Source: CAD feature listing. Evaluate the final solid. Frame: model axes, mm. A direction names the side the tool comes from. Round coordinates to 2 decimals unless told otherwise and drop trailing zeros. Order: outer loops, then holes, each group sorted by start corner. A loop starts at its lowest first (then second) coordinate and runs counter-clockwise, first axis right, second up. Notation, with made-up numbers: (44.5, -5) - (79.5, -5) arc R11 ccw to (79.5, 16) - close; hole circle Ø7 at (-5, -31). An arc over 180 degrees is marked (long way). Use one line per item in the form item = value. Start each with the question number.
Q1. Set-up query: faces 1 (the flat face through (-90, 0, -70)), 2 (the cylindrical face through (-70.02, -0.88, -62.4)), 3 (the cylindrical face through (-109.98, -0.88, 2.39)). Return all of +Z, -Z, +X, -X, +Y, -Y with unobstructed straight access to the full face (end or side cutting, diameter ignored); none if empty.
Q2. Cut plane A-A, the plane x = -90. Return the cut outline in (y, z), and give its area (3 significant figures).
Q3. Cut plane C-C, the plane z = -44.5. Return the cut outline in (x, y), and give its area (3 significant figures).
Q4. Cut plane B-B, the plane y = 0. Return the cut outline in (x, z), and give its area (3 significant figures).
Q5. Cut plane D-D, the plane z = -7.5. Return the cut outline in (x, y).
Q6. Pin query (flat end, axial travel): pin 1 Ø10 at (y, z) = (5, -40) entering from +X; pin 2 Ø10 at (x, z) = (-116.5, -36) entering from +Y; pin 3 Ø5 at (y, z) = (14.5, -40) entering from +X; pin 4 Ø8 at (x, y) = (-152, -29.5) entering from -Z. Return the tip coordinate at first contact, or that it passes through.
Q7. Ray query, line 1 (Z direction, x = -66, y = -24); line 2 (Y direction, x = -119, z = -26); line 3 (X direction, y = 74, z = -24.5). Return the intervals inside material, ascending. Write a range as [from, to].
Autodesk Inventor part; units mm, degrees
ref_plane "YZ Plane" through (0, 0, 0) normal (1, 0, 0) x (0, 1, 0)
ref_plane "XZ Plane" through (0, 0, 0) normal (0, 1, 0) x (-1, 0, 0)
ref_plane "XY Plane" through (0, 0, 0) normal (0, 0, 1) x (1, 0, 0)
ref_plane "РабПлоскость3" through (0.0801, 60, -30) normal (0, 0, 1) x (1, 0, 0)
sketch "Эскиз1" plane through (0.0801, 60, -30) normal (0, 0, 1) x (1, 0, 0)
  line L0 (-0.0801, -60) -> (-90.0801, -60)
  circle A0 centre (-90.0801, -60) radius 87.5
  dimension "d0" = 90
  dimension "d1" = 175
extrude "Выдавливание1" add sketch "Эскиз1" along normal mid plane 50
sketch "Эскиз2" plane through (-90, 0, -5) normal (0, 0, 1) x (1, 0, 0)
  circle A0 centre (0, 0) radius 20
  point P0 (90, 0)
  dimension "d4" = 40
extrude "Выдавливание2" add sketch "Эскиз2" along normal blind 15
sketch "Эскиз3" plane through (-90, 0, -55) normal (0, 0, -1) x (-1, 0, 0)
  circle A0 centre (0, 0) radius 20
  circle A1 centre (0, 0) radius 20
  point P0 (-90, 0)
  dimension "d7" = 40
extrude "Выдавливание3" add sketch "Эскиз3" along normal blind 15
fillet "Сопряжение1" radius 5 1 edges at (-177.5, 0, -5)
fillet "Сопряжение2" radius 5 1 edges at (-177.5, 0, -55)
properties part number "Колесо"
Completed:
q1.face_1 = -Z, +X, -X, +Y, -Y
q1.face_2 = -Z
q1.face_3 = +Z
q2.outline = (-87.5, -50) arc R5 ccw to (-82.5, -55) - (-20, -55) - (-20, -70) - (20, -70) - (20, -55) - (82.5, -55) arc R5 ccw to (87.5, -50) - (87.5, -10) arc R5 ccw to (82.5, -5) - (20, -5) - (20, 10) - (-20, 10) - (-20, -5) - (-82.5, -5) arc R5 ccw to (-87.5, -10) - close
q2.area = 9,930 mm2
q3.outline = circle Ø175 at (-90, 0)
q3.area = 24,100 mm2
q4.outline = (-177.5, -50) arc R5 ccw to (-172.5, -55) - (-110, -55) - (-110, -70) - (-70, -70) - (-70, -55) - (-7.5, -55) arc R5 ccw to (-2.5, -50) - (-2.5, -10) arc R5 ccw to (-7.5, -5) - (-70, -5) - (-70, 10) - (-110, 10) - (-110, -5) - (-172.5, -5) arc R5 ccw to (-177.5, -10) - close
q4.area = 9,930 mm2
q5.outline = circle Ø173.66 at (-90, 0)
q6.pin_1 = -2.5
q6.pin_2 = 84.82
q6.pin_3 = -3.33
q6.pin_4 = -55
q7.line_1 = [-55, -5]
q7.line_2 = [-82.55, 82.55]
q7.line_3 = [-136.69, -43.31]
